Autodesk Fusion 360 part; units mm, degrees
sketch "Bracket Profile" plane through (0, 0, 0) normal (0, 0, 1) x (1, 0, 0) in component "Bracket"
  line L0 (0, 0) -> (0, 25)
  line L1 (0, 25) -> (25, 25)
  line L2 (25, 25) -> (25, 20)
  line L3 (25, 20) -> (5, 0)
  line L4 (5, 0) -> (0, 0)
  dimension "d1" = 5
  dimension "d2" = 25
  dimension "d3" = 25
  dimension "d4" = 5
extrude "Extrude1" add sketch "Bracket Profile" along normal blind 20 in component "Bracket"
sketch "Clearance Hole" plane through (0, 0, 0) normal (-1, 0, 0) x (0, -1, 0) in component "Bracket"
  line L0 (-25, 0) -> (0, 0)
  line L1 (0, 0) -> (0, 20)
  line L2 (0, 20) -> (-25, 20)
  line L3 (-25, 20) -> (-25, 0)
  line L4 (-25, 10) -> (0, 10) construction
  line L5 (-12.5, 20) -> (-12.5, 0) construction
  circle A0 centre (-12.5, 10) radius 2.9
  circle A1 centre (-12.5, 10) radius 4.5
  line L6 (0, 13) -> (-25, 13)
  line L7 (-25, 13) -> (-25, 7)
  line L8 (-25, 7) -> (0, 7)
  line L9 (0, 7) -> (0, 13)
  line L10 (0, 13) -> (-25, 7) construction
  line L11 (-25, 13) -> (0, 7) construction
  line L12 (-6.5, 13) -> (-18.5, 13)
  line L13 (-18.5, 13) -> (-18.5, 7)
  line L14 (-18.5, 7) -> (-6.5, 7)
  line L15 (-6.5, 7) -> (-6.5, 13)
  line L16 (-6.5, 13) -> (-18.5, 7) construction
  line L17 (-18.5, 13) -> (-6.5, 7) construction
  point P0 (-12.5, 10)
  point P1 (-12.5, 10)
  dimension "d9" = 5.8
  dimension "d13" = 9
  dimension "d20" = 25
  dimension "d21" = 6
  dimension "d24" = 12
  dimension "d25" = 6
extrude "Extrude3" add sketch "Clearance Hole" along normal blind 6 contours L3 L6 L7 L8 L13 | L1 L6 L8 L9 L15 in component "Bracket"
hole "Hole1" at (0, 12.5, 10) direction (1, 0, 0) diameter 5.8 end through all in component "Bracket"
extrude "Extrude2" cut sketch "Clearance Hole" against normal through all from surface at -8 contours A1 L8 L14 | A1 L6 L8 L12 L14 | A1 L6 L12 in component "Bracket"
sketch "Shelf stop" plane through (0, 25, 0) normal (0, 1, 0) x (-1, 0, 0) in component "Bracket"
  line L0 (-25, 0) -> (0, 0)
  line L1 (0, 0) -> (0, 7)
  line L2 (0, 7) -> (6, 7)
  line L3 (6, 7) -> (6, 13)
  line L4 (6, 13) -> (0, 13)
  line L5 (0, 13) -> (0, 20)
  line L6 (0, 20) -> (-25, 20)
  line L7 (-25, 20) -> (-25, 0)
  line L8 (0, 20) -> (-25, 20)
  line L9 (-25, 20) -> (-25, 15)
  line L10 (-25, 15) -> (0, 15)
  line L11 (0, 15) -> (0, 20)
  dimension "d28" = 25
  dimension "d29" = 5
extrude "Extrude5" add 1 faces at (10, 15, 0) along direction (0, 0, -1) blind 20 in component "Bracket"
extrude "Extrude4" add sketch "Shelf stop" along normal blind 5 contours L5 L6 L7 L8 L9 L10 L11 in component "Bracket"
sketch "Sketch1" plane through (0, 0, 20) normal (0, 0, 1) x (-1, 0, 0)
  line L0 (-5, 0) -> (-25, -20)
  line L1 (-25, -20) -> (-25, -30)
  line L2 (-25, -30) -> (0, -30)
  line L3 (0, -30) -> (0, 0)
  line L4 (0, 0) -> (-5, 0)
sketch "Latch Lip" plane through (0, 0, 20) normal (0, 0, 1) x (-1, 0, 0) in component "Bracket"
  line L0 (-5, 0) -> (-25, -20)
  line L1 (-25, -20) -> (-25, -30)
  line L2 (-25, -30) -> (0, -30)
  line L3 (0, -30) -> (0, 0)
  line L4 (0, 0) -> (-5, 0)
  line L5 (0, -20) -> (0, -30)
  line L6 (0, -30) -> (-25, -30)
  line L7 (-25, -30) -> (-25, -20)
  line L8 (-25, -20) -> (-22.8787, -17.8787)
  line L9 (-22.8787, -17.8787) -> (0, -17.8787)
  line L10 (0, -20) -> (0, -17.8787)
  dimension "d36" = 3
extrude "Extrude6" add sketch "Latch Lip" along normal blind 5 contours L0 L1 L2 L3 L5 L6 L7 L8 L9 L10 in component "Bracket"
chamfer "Chamfer1" distance 0.8 angle 45 11 edges at (8, 16.6955, 8.3727) (2.5, 0, 20) (13.9393, 8.9393, 20) (25, 30, 20) (12.5, 30, 15) (2.5, 0, -20) (15, 10, -20) (25, 22.5, -20) (25, 25, 25) (12.5, 30, 25) (11.4393, 17.8787, 25) 2 faces at (0, 12.5, -10.9667) (16.6667, 25, 0.6667) in component "Bracket"
chamfer "Chamfer1" distance 0.8 angle 45 8 faces at (-6, 4.3333, 11) (-6, 22.8333, 11) (-2, 2.1667, 13) (-2, 20.6667, 13) (-4, 18.5, 9) (-2, 6.5, 9) (-2, 4.3333, 7) (-2, 22.8333, 7) in component "Bracket"
component "Bracket" placed x (1, 0, 0) y (0, 1, 0) z (0, 0, 1) at (0, 0, 0)
equation "d1 = BracketLipSize"
equation "d2 = ExtrusionSize + BracketLipSize"
equation "d3 = ExtrusionSize + BracketLipSize"
equation "d4 = BracketLipSize"
equation "ExtrusionSize = 20 mm"
equation "BracketLipSize = 5 mm"
equation "d7 = ExtrusionSize"
equation "d9 = ScrewClearanceHole"
equation "ScrewClearanceHole = 5.8 mm"
equation "d11 = ScrewClearanceHole"
equation "d13 = ScrewHeadClearance"
equation "ScrewHeadClearance = 9 mm"
equation "d15 = -ExtrusionSize / 2.5"
equation "Chamfer = 0.8 mm"
equation "d18 = Chamfer"
equation "Tounge = 6 mm"
equation "d20 = ExtrusionSize + BracketLipSize"
equation "d21 = Tounge"
equation "d22 = Tounge"
equation "d24 = NutClearance"
equation "d25 = Tounge"
equation "NutClearance = 12 mm"
equation "d27 = Chamfer"
equation "d28 = ExtrusionSize + BracketLipSize"
equation "d29 = BracketLipSize"
equation "d30 = BracketLipSize"
equation "d32 = ExtrusionSize"
equation "d34 = BracketLipSize"
CAD build for the part. Positions are in the model's coordinates, mm. A direction names the side the tool comes from. Round coordinates to 2 decimals unless told otherwise and drop trailing zeros. Order: outer loops, then holes, each group sorted by start corner. A loop starts at its lowest first (then second) coordinate and runs counter-clockwise, first axis right, second up. Notation, with made-up numbers: (76.25, -2) -> (108.25, -2) arc R20 cw to (108.25, 35) -> close; hole circle Ø10 at (-1.5, 64). An arc over 180 degrees is marked (long way). Write each question's results on one line, items separated by ' | '.
1. Flat gauge pins, fed straight in: P1, Ø3.5, axis at x = -3.5, y = 4, coming from the +Z side; P2, Ø8, axis at y = 13.5, z = 9.5, coming from the +X side; P3, Ø2, axis at y = 15, z = -7, coming from the -X side; P4, Ø5, axis at y = 12.5, z = 10, coming from the -X side. Where does each tip first touch, or does it go through?
Findings below:
P1: stops at z = 13 | P2: stops at x = 22.5 | P3: stops at x = 0 | P4: passes through
2. Pull direction Z, two halves, no side cores. Call faces 1 (the face through (-3, 3, 7)), 2 (the face through (-0.3, 6.3, 12.9)), 3 (the face through (0.3, 25.1, 14.8)), 4 (the face through (-0.1, 24.7, 13.2)): pulls with the +Z half, pulls with the -Z half, needs draft (parallel to the pull), parting line crosses it, or undercut.
Findings below:
face 1: pulls with the -Z half | face 2: pulls with the +Z half | face 3: undercut | face 4: undercut
3. Wall check: line 1 along Y through (x, z) = (11.5, 10); line 2 along Z through (x, y) = (5, 12); line 3 along X through (y, z) = (2, 18). Give the ranges that are in metal, low to high. Write a range as [from, to].
Findings below:
line 1: y = [6.5, 8], [17, 25] | line 2: z = [-20, 7.14], [12.86, 20] | line 3: x = [0, 7]
4. Cut at C-C (y = 12.5). Give the cut face in (x, z), plus the area to 3 significant figures.
Findings below:
outline: (0, -19.2) -> (0.8, -20) -> (16.37, -20) -> (17.5, -19.2) -> (17.5, 5.5) -> (8.8, 5.5) -> (8, 6.3) -> (8, 7.1) -> (0.8, 7.1) -> (0, 6.3) -> close; (0, 13.7) -> (0.8, 12.9) -> (8, 12.9) -> (8, 13.7) -> (8.8, 14.5) -> (17.5, 14.5) -> (17.5, 19.2) -> (16.37, 20) -> (0.8, 20) -> (0, 19.2) -> close | area: 567 mm²
5. Cut at B-B (x = 1.5). Give the cut face in (y, z).
Findings below:
outline: (0, -19.2) -> (0.8, -20) -> (24.2, -20) -> (25, -19.2) -> (25, 14.2) -> (25.8, 15) -> (29.2, 15) -> (30, 15.8) -> (30, 24.2) -> (29.2, 25) -> (18.68, 25) -> (17.88, 24.2) -> (17.88, 20) -> (0.8, 20) -> (0, 19.2) -> close; hole circle Ø5.8 at (12.5, 10)
6. Cut at D-D (z = -10.5). Give the cut face in (x, y), plus the area to 3 significant figures.
Findings below:
outline: (0, 0.8) -> (0.8, 0) -> (5, 0) -> (25, 20) -> (25, 24.2) -> (24.2, 25) -> (0.8, 25) -> (0, 24.2) -> close | area: 424 mm²
7. 3-axis set-ups, long thin cutter, end or side, ignore diameter. For faces 5 (the face through (-3, 3, 13)), 6 (the face through (-3, 6.5, 10)), 7 (the face through (14, 17, 10)): which of +Z, -Z, +X, -X, +Y, -Y reach the whole face in a straight line?
Findings below:
face 5: +Z, -X, +Y, -Y | face 6: +Z, -Z, -X | face 7: +X
8. Cut at A-A (z = 10). Give the cut face in (x, y), plus the area to 3 significant figures.
Findings below:
outline: (-6, 0.8) -> (-5.2, 0) -> (5, 0) -> (13, 8) -> (8.8, 8) -> (8, 8.8) -> (8, 9.6) -> (0.8, 9.6) -> (0, 8.8) -> (0, 7.3) -> (-0.8, 6.5) -> (-5.2, 6.5) -> (-6, 5.7) -> close; (-6, 19.3) -> (-5.2, 18.5) -> (-0.8, 18.5) -> (0, 17.7) -> (0, 16.2) -> (0.8, 15.4) -> (8, 15.4) -> (8, 16.2) -> (8.8, 17) -> (22, 17) -> (25, 20) -> (25, 24.2) -> (24.2, 25) -> (-5.2, 25) -> (-6, 24.2) -> close | area: 370 mm²
